Model file for the job. Use its own axes, mm. A direction names the side the tool comes from. Give positions to 0.01 mm unless a question says otherwise; leave off trailing zeros. Loops run counter-clockwise (first coordinate to the right, second up) from the corner with the lowest first, then second, coordinate; pieces in that order, holes last. Notation, with made-up numbers: (-4, 61.25) - (31, 61.25) arc R34 cw to (31, 100.25) - close; hole circle Ø3 at (27, -35). An arc over 180 degrees is marked (long way). Use a Markdown table: item, result.
from build123d import *

# Parameters (mm, degrees)
F0_W     = 44.45
F0_H     = 12.7
F1_DEPTH = 3.175
F3_DEPTH = 3.176


with BuildPart() as f1:
    # F0 (on Top) → F1 (new body)
    with BuildSketch(Plane.XY):
        with Locations((-1.5875, 0)):
            Rectangle(F0_W, F0_H)
    extrude(amount=F1_DEPTH)

    # F2 (on Top) → F3 (cut, through all)
    with BuildSketch(Plane.XY):
        with BuildLine():
            ThreePointArc((8.647452, 3.529976), (7.582524, 3.884952), (7.227548, 2.820024))
            Line((7.227548, 2.820024), (10.402548, -3.529976))
            ThreePointArc((10.402548, -3.529976), (11.467476, -3.884952), (11.822452, -2.820024))
            Line((11.822452, -2.820024), (8.647452, 3.529976))
        make_face()
    extrude(amount=F3_DEPTH, mode=Mode.SUBTRACT)


solid = f1.part
(1) Mould opens along Y. For faces 1 (the flat face through (-2, -6.35, 2)), 2 (the flat face through (-23.812, 0, 2)), 3 (the flat face through (8.793, -0.311, 1.565)) say: pulls with the +Y half, pulls with the -Y half, needs draft (parallel to the pull), parting line crosses it, or undercut.
Computed:
| item | result |
|---|---|
| face 1 | pulls with the -Y half |
| face 2 | needs draft |
| face 3 | undercut |
(2) Slice it at A-A, the plane y = -1.25. Write the cut outline in (x, z) (1 decimal), plus the area to 3 significant figures.
Computed:
| item | result |
|---|---|
| outline | (-23.8, 0) - (9.3, 0) - (9.3, 3.2) - (-23.8, 3.2) - close; (11, 0) - (20.6, 0) - (20.6, 3.2) - (11, 3.2) - close |
| area | 135 mm² |
(3) 3-axis set-ups, long thin cutter, end or side, ignore diameter. For faces 4 (the flat face through (10.257, 0.311, 1.565)), 5 (the flat face through (-2, 0, 3.175)): which of +Z, -Z, +X, -X, +Y, -Y reach the whole face in a straight line?
Computed:
| item | result |
|---|---|
| face 4 | +Z, -Z |
| face 5 | +Z, +X, -X, +Y, -Y |
(4) Drill centre lines: probe 1 along Y at (x, z) = (8, 2.35); probe 2 along X at (y, z) = (-2.75, 2.75); probe 3 along X at (y, z) = (-2, 0.5). Where is each one in solid material? Low to high. Write a range as [from, to].
Computed:
| item | result |
|---|---|
| probe 1 | [-6.35, 1.28], [3.97, 6.35] |
| probe 2 | [-23.81, 10.01], [11.79, 20.64] |
| probe 3 | [-23.81, 9.64], [11.41, 20.64] |
